Verification items for the finished model (mm, model axes). A direction names the side the tool comes from. Coordinates: 2 decimals unless noted, no trailing zeros. Write each loop counter-clockwise with the first axis right and the second up, starting at its lowest first coordinate (ties: lowest second). Pieces come first, ordered by that corner, then holes. Notation, with made-up numbers: (42.25, 62) -> (48.25, 62) arc R9 ccw to (48.25, 71) -> close; hole circle Ø8 at (27.25, 26.25). An arc over 180 degrees is marked (long way). Write item = value, one per line. Start each with the question number.
(1) Gauge pin test, flat ends, axial feed: pin 1 Ø2 at (x, z) = (24.5, 25) entering from +Y; pin 2 Ø4 at (x, z) = (-27.5, 39.5) entering from -Y; pin 3 Ø1 at (x, y) = (18.5, 6) entering from +Z. Record the tip position at first contact, or that the pin passes through.
(2) Material ranges on probe 1 along X at (y, z) = (9, 25); probe 2 along X at (y, z) = (5.75, -25.5); probe 3 along X at (y, z) = (2.15, -39.5), recorded low to high. Write a range as [from, to].
(3) Set-up check for faces 1 (the face through (27, 7, 25)), 2 (the face through (29.6, 1.77, -41.64)): record each of +Z, -Z, +X, -X, +Y, -Y from which the full face is reachable in a straight line by a thin tool's end or side.
(4) Mould release check, pull along Z, two halves, no side actions. Record for faces 3 (the face through (-8, 3.5, -26)), 4 (the face through (0, 2, 42.5)), 5 (the face through (-29.64, 1.77, -41.6)): released by +Z, released by -Z, zero draft, split by the parting line, or undercut.
(5) Section check C-C (z = -25.5). Record the cut outline in (x, y).
(6) Section check A-A (y = 7.5). Record the cut outline in (x, z), plus the area to 3 significant figures.
(7) Section check B-B (x = -8.5). Record the cut outline in (y, z).
(8) Section check D-D (x = -16). Record the cut outline in (y, z), plus the area to 4 significant figures.
```python
from build123d import *

# Parameters (mm, degrees)
SKETCH1_W           = 61
SKETCH1_H           = 85
BOSS_EXTRUDE1_DEPTH = 3.5
SKETCH2_R           = 1.5
CUT_EXTRUDE1_DEPTH  = 3.5
SKETCH3_R           = 2.5
BOSS_EXTRUDE2_DEPTH = 7.5
SKETCH4_R           = 1.35
CUT_EXTRUDE2_DEPTH  = 7.5
FILLET1_R           = 3


with BuildPart() as part:
    # Sketch1 → Boss-Extrude1 (new body)
    with BuildSketch(Plane(origin=(0, 0, 0), x_dir=(1, 0, 0), z_dir=(0, 1, 0))):
        Rectangle(SKETCH1_W, SKETCH1_H)
    extrude(amount=BOSS_EXTRUDE1_DEPTH)

    # Sketch2 → Cut-Extrude1 (cut)
    with BuildSketch(Plane(origin=(0, 3.5, 0), x_dir=(1, 0, 0), z_dir=(0, 1, 0))):
        with Locations(Location((-27.5, 39.5, 0), (0, 0, 270))):
            Circle(SKETCH2_R)
        with Locations(Location((27.5, 39.5, 0), (0, 0, 270))):
            Circle(SKETCH2_R)
        with Locations(Location((-27.5, -39.5, 0), (0, 0, 270))):
            Circle(SKETCH2_R)
        with Locations(Location((27.5, -39.5, 0), (0, 0, 270))):
            Circle(SKETCH2_R)
    extrude(amount=-CUT_EXTRUDE1_DEPTH, mode=Mode.SUBTRACT)

    # Sketch3 → Boss-Extrude2 (add)
    with BuildSketch(Plane(origin=(0, 3.5, 0), x_dir=(1, 0, 0), z_dir=(0, 1, 0))):
        with Locations(Location((-24.5, -25, 0), (0, 0, 270))):
            Circle(SKETCH3_R)
        with Locations(Location((24.5, -25, 0), (0, 0, 270))):
            Circle(SKETCH3_R)
        with Locations(Location((19.5, 25.5, 0), (0, 0, 270))):
            Circle(SKETCH3_R)
        with Locations(Location((-8.5, 25.5, 0), (0, 0, 270))):
            Circle(SKETCH3_R)
    extrude(amount=BOSS_EXTRUDE2_DEPTH)

    # Sketch4 → Cut-Extrude2 (cut)
    with BuildSketch(Plane(origin=(0, 11, 0), x_dir=(1, 0, 0), z_dir=(0, 1, 0))):
        with Locations(Location((-8.5, 25.5, 0), (0, 0, 270))):
            Circle(SKETCH4_R)
        with Locations(Location((19.5, 25.5, 0), (0, 0, 270))):
            Circle(SKETCH4_R)
        with Locations(Location((-24.5, -25, 0), (0, 0, 270))):
            Circle(SKETCH4_R)
        with Locations(Location((24.5, -25, 0), (0, 0, 270))):
            Circle(SKETCH4_R)
    extrude(amount=-CUT_EXTRUDE2_DEPTH, mode=Mode.SUBTRACT)

    # Fillet1
    fillet1_edges = [part.edges().sort_by_distance(p)[0] for p in [
        (30.5, 1.75, 42.5),
        (-30.5, 1.75, 42.5),
        (-30.5, 1.75, -42.5),
        (30.5, 1.75, -42.5),
    ]]
    fillet(fillet1_edges, radius=FILLET1_R)


solid = part.part
```
Response:
q1.pin_1 = 3.5
q1.pin_2 = 0
q1.pin_3 = -23.05
q2.probe_1 = [-27, -25.85], [-23.15, -22], [22, 23.15], [25.85, 27]
q2.probe_2 = [-11, -9.85], [-7.15, -6], [17, 18.15], [20.85, 22]
q2.probe_3 = [-30.5, -29], [-26, 26], [29, 30.5]
q3.face_1 = +Y
q3.face_2 = -Z, +X, +Y, -Y
q4.face_3 = undercut
q4.face_4 = released by +Z
q4.face_5 = released by -Z
q5.outline = (-30.5, 0) -> (30.5, 0) -> (30.5, 3.5) -> (22, 3.5) -> (22, 11) -> (20.85, 11) -> (20.85, 3.5) -> (18.15, 3.5) -> (18.15, 11) -> (17, 11) -> (17, 3.5) -> (-6, 3.5) -> (-6, 11) -> (-7.15, 11) -> (-7.15, 3.5) -> (-9.85, 3.5) -> (-9.85, 11) -> (-11, 11) -> (-11, 3.5) -> (-30.5, 3.5) -> close
q6.outline = circle Ø5 at (-24.5, 25); circle Ø5 at (-8.5, -25.5); circle Ø5 at (19.5, -25.5); circle Ø5 at (24.5, 25); hole circle Ø2.7 at (-24.5, 25); hole circle Ø2.7 at (-8.5, -25.5); hole circle Ø2.7 at (19.5, -25.5); hole circle Ø2.7 at (24.5, 25)
q6.area = 55.6 mm2
q7.outline = (0, -42.5) -> (3.5, -42.5) -> (3.5, -28) -> (11, -28) -> (11, -26.85) -> (3.5, -26.85) -> (3.5, -24.15) -> (11, -24.15) -> (11, -23) -> (3.5, -23) -> (3.5, 42.5) -> (0, 42.5) -> close
q8.outline = (0, -42.5) -> (3.5, -42.5) -> (3.5, 42.5) -> (0, 42.5) -> close
q8.area = 297.5 mm2
